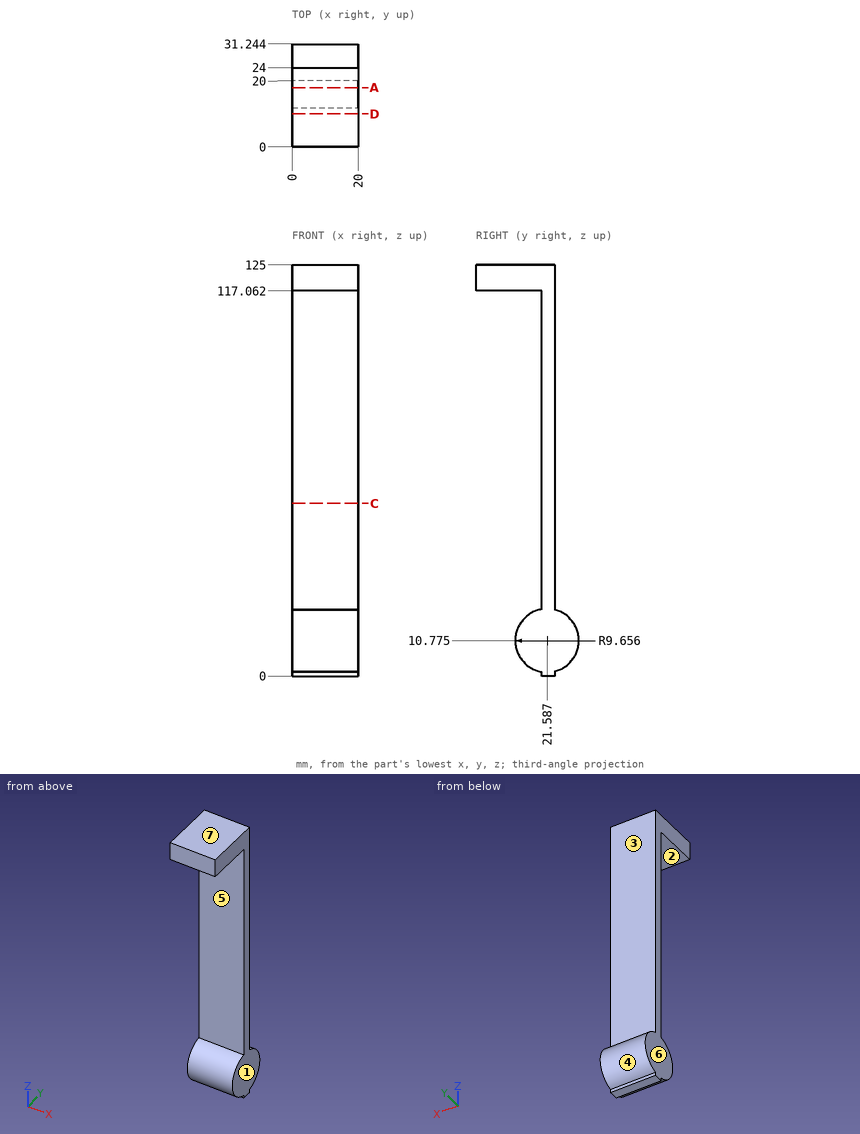
Here's the drawing with two shaded views (mm, measured from the low corner). I have some questions. A direction names the side the tool comes from. Coordinates: 2 decimals unless noted, no trailing zeros. Loops run counter-clockwise (first coordinate to the right, second up) from the corner with the lowest first, then second, coordinate; pieces in that order, holes last. Notation, with made-up numbers: (-9, 23) -> (6, 23) arc R22 ccw to (6, 33) -> close; hole circle Ø4 at (12.25, -7.75). An arc over 180 degrees is marked (long way). Put each result on its own line as item: value. Start each with the question number.
Q1. If I drill on line 1 (Y direction, x = 9.75, z = 54.5); line 2 (Z direction, x = 4.25, y = 9.5); line 3 (Z direction, x = 11.75, y = 18), over which ranges is the centre line in solid material (lowest first)? Write a range as [from, to].
Q2. Thinking about a two-plate mould opening in Z: for the marked faces 4, 5, 6 and 7, which applies, pulls with the +Z half, pulls with the -Z half, needs draft (parallel to the pull), parting line crosses it, or undercut?
Q3. I'm going to push flat-ended pins straight in: P1, Ø1.5, axis at x = 9, z = 38.5, coming from the -Y side; P2, Ø1.5, axis at x = 10.5, z = 75, coming from the +Y side; P3, Ø10, axis at x = 16, y = 14.5, coming from the -Z side. Where does each tip first touch, or does it pass through?
Q4. I want a section at C-C (z = 52.5). Write out the boundary of the cut face in (x, y).
Q5. For the marked faces 1, 2 and 3, which set-ups out of +Z, -Z, +X, -X, +Y, -Y let a thin tool reach every point of the face, with its end or its side?
Q6. I want a section at A-A (y = 18). Write out the boundary of the cut face in (x, z).
Q7. I want a section at D-D (y = 10). Write out the boundary of the cut face in (x, z), plus the area to 3 significant figures.
Taken from the geometry:
1. line 1: y = [20, 24]
1. line 2: z = [117.06, 125]
1. line 3: z = [1.81, 19.74], [117.06, 125]
2. face 4: parting line crosses it
2. face 5: undercut
2. face 6: needs draft
2. face 7: pulls with the +Z half
3. P1: stops at y = 20
3. P2: stops at y = 24
3. P3: stops at z = 1.35
4. outline: (0, 20) -> (20, 20) -> (20, 24) -> (0, 24) -> close
5. face 1: +Z, -Z, +X, +Y, -Y
5. face 2: +X, -X, -Y
5. face 3: +Z, +X, -X, +Y
6. outline: (0, 1.81) -> (20, 1.81) -> (20, 19.74) -> (0, 19.74) -> close; (0, 117.06) -> (20, 117.06) -> (20, 125) -> (0, 125) -> close
7. outline: (0, 117.06) -> (20, 117.06) -> (20, 125) -> (0, 125) -> close
7. area: 159 mm2
